```python
from build123d import *

# Parameters (mm, degrees)
ESQUISSE4_W             = 75
ESQUISSE4_H             = 56
BOSS_EXTRU_2_DEPTH      = 18
ESQUISSE5_R             = 6
ENL_V_MAT_EXTRU_3_DEPTH = 51.142297514
ESQUISSE6_W             = 32
ESQUISSE6_H             = 6
ENL_V_MAT_EXTRU_4_DEPTH = 83.054859698
ESQUISSE9_R             = 18
ESQUISSE9_R_2           = 11
BOSS_EXTRU_3_DEPTH      = 25
BOSS_EXTRU_6_REACH      = 99.32
BOSS_EXTRU_6_END_RADIUS = 18
ESQUISSE10_W            = 12
ESQUISSE10_H            = 25
BOSS_EXTRU_7_DEPTH      = 6


with BuildPart() as part:
    # Esquisse4 → Boss.-Extru.2 (new body)
    with BuildSketch(Plane(origin=(0, 0, 0), x_dir=(1, 0, 0), z_dir=(0, 1, 0))):
        Rectangle(ESQUISSE4_W, ESQUISSE4_H)
    extrude(amount=BOSS_EXTRU_2_DEPTH)

    # Esquisse5 → Enlèv. mat.-Extru.3 (cut, through all)
    with BuildSketch(Plane(origin=(0, 18, 0), x_dir=(1, 0, 0), z_dir=(0, 1, 0))):
        with Locations(Location((22.5, 0, 0), (0, 0, 270))):
            Circle(ESQUISSE5_R)
    enl_v_mat_extru_3 = extrude(amount=-ENL_V_MAT_EXTRU_3_DEPTH, mode=Mode.SUBTRACT)

    # Symétrie1: Enlèv. mat.-Extru.3 across plane
    add(enl_v_mat_extru_3.mirror(Plane(origin=(0, 0, 0), x_dir=(0, 0, 1), z_dir=(1, 0, 0))), mode=Mode.SUBTRACT)

    # Esquisse6 → Enlèv. mat.-Extru.4 (cut, through all)
    with BuildSketch(Plane(origin=(37.5, 0, 0), x_dir=(0, 0, -1), z_dir=(1, 0, 0))):
        with Locations((0, 3)):
            Rectangle(ESQUISSE6_W, ESQUISSE6_H)
    extrude(amount=-ENL_V_MAT_EXTRU_4_DEPTH, mode=Mode.SUBTRACT)



with BuildPart() as body_2:
    # Esquisse9 → Boss.-Extru.3 (new body)
    with BuildSketch(Plane(origin=(0, 63, 0), x_dir=(-1, 0, 0), z_dir=(0, -1, 0))):
        with Locations(Location((0, 72, 0), (0, 0, 90))):
            Circle(ESQUISSE9_R)
        with Locations(Location((0, 72, 0), (0, 0, 90))):
            Circle(ESQUISSE9_R_2, mode=Mode.SUBTRACT)
    extrude(amount=BOSS_EXTRU_3_DEPTH)

    # Boss.-Extru.6: up to this cylinder (the profile starts outside it)
    boss_extru_6_end = Plane(origin=(0, 50.5, -72), z_dir=(0, 1, 0)) * Cylinder(BOSS_EXTRU_6_END_RADIUS, 235.64, mode=Mode.PRIVATE)
    # Esquisse10 → Boss.-Extru.6 (add, up to the surface)
    with BuildSketch(Plane.XY.offset(-36), mode=Mode.PRIVATE) as boss_extru_6_sk1:
        with Locations((0, 50.5)):
            Rectangle(ESQUISSE10_W, ESQUISSE10_H)
    boss_extru_6_tool1 = extrude(boss_extru_6_sk1.sketch, amount=-BOSS_EXTRU_6_REACH, mode=Mode.PRIVATE) - boss_extru_6_end
    add(boss_extru_6_tool1.solids().sort_by_distance((0, 50.5, -36))[0])


with BuildPart() as part_1:
    add(part.part)

    add(body_2.part)  # Boss.-Extru.7 merges body 2
    # Esquisse11 → Boss.-Extru.7 (add, symmetric)
    with BuildSketch(Plane(origin=(0, 0, 0), x_dir=(0, 0, -1), z_dir=(1, 0, 0))):
        Polygon((36, 63), (-28, 18), (28, 18), (28, 0), (55.029437252, 38), (36, 38), align=None)
    extrude(amount=BOSS_EXTRU_7_DEPTH, both=True)


solid = part_1.part
```
Work out the finished part from the listing and answer in its coordinate system (mm). A direction names the side the tool comes from. Round coordinates to 2 decimals unless told otherwise and drop trailing zeros. Write each loop counter-clockwise with the first axis right and the second up, starting at its lowest first coordinate (ties: lowest second). Pieces come first, ordered by that corner, then holes.
1) Which of the six approach directions +Z, -Z, +X, -X, +Y, -Y give full straight-line access (tool end or side, diameter ignored) to faces 4 (the face through (1, 3, 16)), 5 (the face through (22, 18, -7)), 6 (the face through (-8, 38, -80))?
2) Consider probe 1 along X at (y, z) = (13, 0); probe 2 along X at (y, z) = (31, -10); probe 3 along Z at (x, y) = (-22, 15). Determine where each line is inside the solid, lowest interval first.
3) Determine the mould class of faces 1 (the face through (17.177, 12.084, 2.769)), 2 (the face through (-22, 9, -28)), 3 (the face through (-8, 63, -63)) for opening direction Z: pulls with the +Z half, pulls with the -Z half, needs draft (parallel to the pull), parting line crosses it, or undercut.
4) Flat-ended cylindrical pins translate along their axes: P1, Ø5.5, axis at x = -15, y = 11.5, coming from the -Z side; P2, Ø12, axis at y = 28.5, z = -2, coming from the -X side; P3, Ø1, axis at x = -2.5, z = -7, coming from the +Y side; P4, Ø12, axis at x = 9.5, z = -36.5, coming from the +Y side. Find the tip coordinate at first contact, or state that the pin passes through.
5) A cutting plane is placed at D-D on x = 0. Determine the outline of the cut face in (y, z), and give its area (3 significant figures).
6) A cutting plane is placed at A-A on x = 22.5. Determine the outline of the cut face in (y, z), and give its area (3 significant figures).
7) A cutting plane is placed at C-C on y = 9. Determine the outline of the cut face in (x, z).
8) A cutting plane is placed at B-B on z = -72. Determine the outline of the cut face in (x, y), and give its area (3 significant figures).
Entries:
1. face 4: +X, -X, -Y
1. face 5: +Z, -Z, +X, +Y
1. face 6: -Z, +X, -X, -Y
2. probe 1: x = -37.5 to -28.5, -16.5 to 16.5, 28.5 to 37.5
2. probe 2: x = -6 to 6
2. probe 3: z = -28 to -5.98, 5.98 to 28
3. face 1: undercut
3. face 2: pulls with the -Z half
3. face 3: needs draft
4. P1: stops at z = -28
4. P2: stops at x = -6
4. P3: stops at y = 42.96
4. P4: stops at y = 63
5. outline: (0, -28) - (38, -55.03) - (38, -61) - (63, -61) - (63, -36) - (18, 28) - (0, 28) - (0, 16) - (6, 16) - (6, -16) - (0, -16) - close; (38, -90) - (63, -90) - (63, -83) - (38, -83) - close
5. area: 3,410 mm2
6. outline: (0, -28) - (18, -28) - (18, -6) - (6, -6) - (6, -16) - (0, -16) - close; (0, 16) - (6, 16) - (6, 6) - (18, 6) - (18, 28) - (0, 28) - close
6. area: 672 mm2
7. outline: (-37.5, -28) - (-6, -28) - (-6, -34.4) - (6, -34.4) - (6, -28) - (37.5, -28) - (37.5, 28) - (-37.5, 28) - close; hole circle Ø12 at (-22.5, 0); hole circle Ø12 at (22.5, 0)
8. outline: (-18, 38) - (-11, 38) - (-11, 63) - (-18, 63) - close; (11, 38) - (18, 38) - (18, 63) - (11, 63) - close
8. area: 350 mm2
